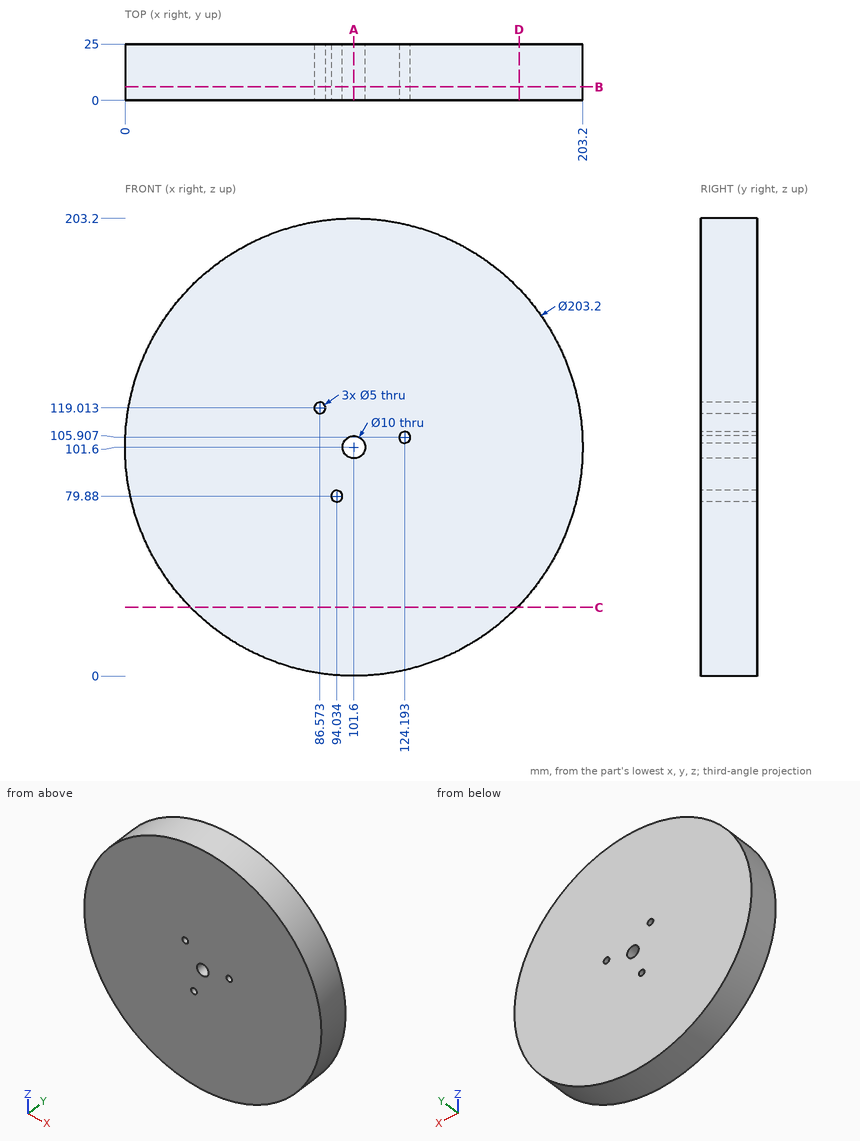
Geometry check sheet. Reference: drawing and pictorial views, mm from the part's lowest x, y, z. Round coordinates to 2 decimals unless told otherwise and drop trailing zeros. Loops run counter-clockwise (first coordinate to the right, second up) from the corner with the lowest first, then second, coordinate; pieces in that order, holes last. Notation, with made-up numbers: (-33, 76.5) - (-11, 76.5) arc R30 ccw to (-11, 101.5) - close; hole circle Ø7 at (22.5, 46). An arc over 180 degrees is marked (long way). Write item = value, one per line. Start each with the question number.
Q1. Section check B-B (y = 6). Record the boundary of the cut face in (x, z), plus the area to 3 significant figures.
Q2. Thickness scan on L1, parallel to X at y = 5.5, z = 101.6; L2, parallel to X at y = 2.75, z = 100; L3, parallel to Z at x = 92.5, y = 23.75 (1 decimal). Record the ranges inside material, lowest first.
Q3. Depth check by flat-ended pin: P1, Ø8, axis at x = 151, y = 15.5, coming from the -Z side; P2, Ø2, axis at x = 108.5, y = 10, coming from the -Z side; P3, Ø8, axis at x = 144.5, y = 15, coming from the +Z side. Enter the tip coordinate at first touch or a pass-through.
Q4. Section check A-A (x = 101.6). Record the boundary of the cut face in (y, z).
Q5. Section check D-D (x = 175). Record the boundary of the cut face in (y, z), plus the area to 3 significant figures.
Q6. Section check C-C (z = 30.5). Record the boundary of the cut face in (x, y), plus the area to 3 significant figures.
Derived:
q1.outline = circle Ø203.2 at (101.6, 101.6); hole circle Ø5 at (86.57, 119.01); hole circle Ø5 at (94.03, 79.88); hole circle Ø10 at (101.6, 101.6); hole circle Ø5 at (124.19, 105.91)
q1.area = 32,300 mm^2
q2.L1 = 0 to 96.6, 106.6 to 203.2
q2.L2 = 0.01 to 96.86, 106.34 to 203.19
q2.L3 = 0.4 to 77.9, 81.9 to 202.8
q3.P1 = 10.71
q3.P2 = 0.17
q3.P3 = 195.46
q4.outline = (0, 0) - (25, 0) - (25, 96.6) - (0, 96.6) - close; (0, 106.6) - (25, 106.6) - (25, 203.2) - (0, 203.2) - close
q5.outline = (0, 31.35) - (25, 31.35) - (25, 171.85) - (0, 171.85) - close
q5.area = 3,510 mm^2
q6.outline = (29.02, 0) - (174.18, 0) - (174.18, 25) - (29.02, 25) - close
q6.area = 3,630 mm^2
